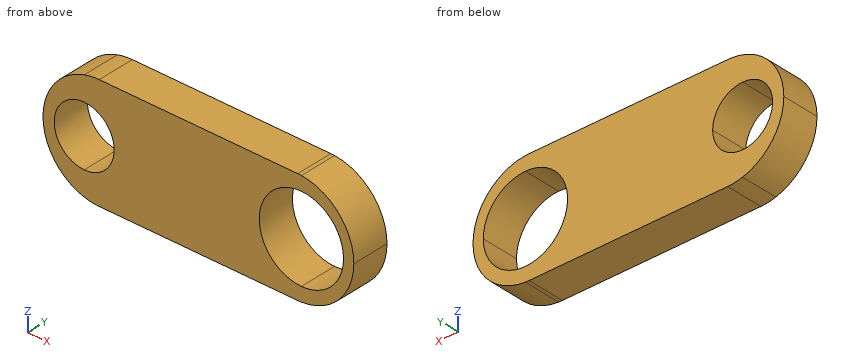
```python
from build123d import *

# Parameters (mm, degrees)
F1_DEPTH = 10


with BuildPart() as f1:
    # F0 (on Front) → F1 (new body)
    with BuildSketch(Plane.XZ):
        with BuildLine():
            Line((-26.5, -15), (26.5, -15))
            ThreePointArc((26.5, -15), (27.000278, -14.991655), (27.5, -14.96663))
            Line((27.5, -14.96663), (27.5, -11.25))
            ThreePointArc((27.5, -11.25), (16.25, 0), (27.5, 11.25))
            Line((27.5, 11.25), (27.5, 14.96663))
            ThreePointArc((27.5, 14.96663), (27.000278, 14.991655), (26.5, 15))
            Line((26.5, 15), (-26.5, 15))
            ThreePointArc((-26.5, 15), (-28.518355, 14.863588), (-30.5, 14.456832))
            Line((-30.5, 14.456832), (-30.5, 8))
            ThreePointArc((-30.5, 8), (-24.843146, 5.656854), (-22.5, 0))
            ThreePointArc((-22.5, 0), (-24.843146, -5.656854), (-30.5, -8))
            Line((-30.5, -8), (-30.5, -14.456832))
            ThreePointArc((-30.5, -14.456832), (-28.518355, -14.863588), (-26.5, -15))
        make_face()
        with BuildLine():
            Line((27.5, -11.25), (27.5, -14.96663))
            ThreePointArc((27.5, -14.96663), (37.454451, -10.246951), (41.5, 0))
            ThreePointArc((41.5, 0), (37.454451, 10.246951), (27.5, 14.96663))
            Line((27.5, 14.96663), (27.5, 11.25))
            ThreePointArc((27.5, 11.25), (35.454951, 7.954951), (38.75, 0))
            ThreePointArc((38.75, 0), (35.454951, -7.954951), (27.5, -11.25))
        make_face()
        with BuildLine():
            ThreePointArc((-41.5, 0), (-38.437336, -9.082951), (-30.5, -14.456832))
            Line((-30.5, -14.456832), (-30.5, -8))
            ThreePointArc((-30.5, -8), (-38.5, 0), (-30.5, 8))
            Line((-30.5, 8), (-30.5, 14.456832))
            ThreePointArc((-30.5, 14.456832), (-38.437336, 9.082951), (-41.5, 0))
        make_face()
    extrude(amount=F1_DEPTH)


solid = f1.part
```
The model under review builds one solid part; all positions refer to its coordinate system, in mm. Round coordinates to 2 decimals unless told otherwise and drop trailing zeros. Loops run counter-clockwise (first coordinate to the right, second up) from the corner with the lowest first, then second, coordinate; pieces in that order, holes last. Notation, with made-up numbers: (-36.75, 62) -> (5.25, 62) arc R27 ccw to (5.25, 97) -> close; hole circle Ø3 at (81, 83.5). An arc over 180 degrees is marked (long way). Answer in a Markdown table with one row per item.
1) Wall thickness on line 1 along X through (y, z) = (-5.25, -6.5); line 2 along X through (y, z) = (-1.25, -3); line 3 along X through (y, z) = (-8.5, 9): over which ranges is each line inside the solid? List them lowest first.
Taken from the geometry:
| item | result |
|---|---|
| line 1 | x = -40.02 to -35.16, -25.84 to 18.32, 36.68 to 40.02 |
| line 2 | x = -41.2 to -37.92, -23.08 to 16.66, 38.34 to 41.2 |
| line 3 | x = -38.5 to 20.75, 34.25 to 38.5 |
2) Consider section D-D, the plane z = -1.5. Write out the cut boundary in (x, y).
Taken from the geometry:
| item | result |
|---|---|
| outline | (-41.42, -10) -> (-38.36, -10) -> (-38.36, 0) -> (-41.42, 0) -> close; (-22.64, -10) -> (16.35, -10) -> (16.35, 0) -> (-22.64, 0) -> close; (38.65, -10) -> (41.42, -10) -> (41.42, 0) -> (38.65, 0) -> close |
3) Consider section A-A, the plane z = -5. Write out the cut boundary in (x, y) (3 decimals).
Taken from the geometry:
| item | result |
|---|---|
| outline | (-40.642, -10) -> (-36.745, -10) -> (-36.745, 0) -> (-40.642, 0) -> close; (-24.255, -10) -> (17.422, -10) -> (17.422, 0) -> (-24.255, 0) -> close; (37.578, -10) -> (40.642, -10) -> (40.642, 0) -> (37.578, 0) -> close |
4) Consider section C-C, the plane x = -33.5. Write out the cut boundary in (y, z).
Taken from the geometry:
| item | result |
|---|---|
| outline | (-10, -13.27) -> (0, -13.27) -> (0, -7.42) -> (-10, -7.42) -> close; (-10, 7.42) -> (0, 7.42) -> (0, 13.27) -> (-10, 13.27) -> close |
5) For pin 1 Ø6 at (y, z) = (-5.5, 6) entering from +X; pin 2 Ø1 at (y, z) = (-8, 9.5) entering from +X, all flat-tipped, find the tip position at first contact; note any pin that passes through.
Taken from the geometry:
| item | result |
|---|---|
| pin 1 | stops at x = 41.2 |
| pin 2 | stops at x = 38.5 |
6) Consider section B-B, the plane y = -3.25. Write out the cut boundary in (x, z).
Taken from the geometry:
| item | result |
|---|---|
| outline | (-41.5, 0) arc R15 ccw to (-30.5, -14.46) arc R15 ccw to (-26.5, -15) -> (26.5, -15) arc R15 ccw to (27.5, -14.97) arc R15 ccw to (27.5, 14.97) arc R15 ccw to (26.5, 15) -> (-26.5, 15) arc R15 ccw to (-30.5, 14.46) arc R15 ccw to start; hole (-30.5, -8) arc R8 ccw to (-22.5, 0) arc R8 ccw (long way) to start; hole (27.5, -11.25) arc R11.25 ccw to (38.75, 0) arc R11.25 ccw (long way) to start |
